Can you work these out from the model? Positions are in its coordinate system, mm. A direction names the side the tool comes from. Round coordinates to 2 decimals unless told otherwise and drop trailing zeros. Loops run counter-clockwise (first coordinate to the right, second up) from the corner with the lowest first, then second, coordinate; pieces in that order, holes last. Notation, with made-up numbers: M 58,69 L 105,69 A25 cw 105,95 Z; hole C 71,-31.75 d5. An arc over 180 degrees is marked long. Return JSON: item names as keys, results as strings.
```python
from build123d import *

# Parameters (mm, degrees)
IZIM1_R                     = 12.2
Y_KSEKLIK_EKSTR_ZYON1_DEPTH = 30.8
RADYUS1_R                   = 0.5
IZIM2_R                     = 12.2
Y_KSEKLIK_EKSTR_ZYON2_DEPTH = 21
IZIM3_R                     = 3.5
Y_KSEKLIK_EKSTR_ZYON3_DEPTH = 2.5
IZIM4_R                     = 2
Y_KSEKLIK_EKSTR_ZYON4_DEPTH = 9
IZIM5_R                     = 1
KES_EKSTR_ZYON1_DEPTH       = 10
IZIM6_R                     = 1.5
IZIM6_R_2                   = 1.3
KES_EKSTR_ZYON2_DEPTH       = 1
KES_EKSTR_ZYON3_START       = -8
KES_EKSTR_ZYON3_DEPTH       = 8
IZIM9_R                     = 3.25
Y_KSEKLIK_EKSTR_ZYON5_DEPTH = 1
IZIM10_R                    = 0.75
Y_KSEKLIK_EKSTR_ZYON6_DEPTH = 15
IZIM11_W                    = 0.852537123
IZIM11_H                    = 3
Y_KSEKLIK_EKSTR_ZYON7_DEPTH = 4
IZIM12_R                    = 0.75
KES_EKSTR_ZYON4_DEPTH       = 4
PAH1_SIZE                   = 1


with BuildPart() as part:
    # izim1 → Y_kseklik-Ekstr_zyon1 (new body)
    with BuildSketch(Plane.XY):
        with Locations(Location((-41.143471688, 10.161406423, 0), (0, 0, 180))):
            Circle(IZIM1_R)
    extrude(amount=Y_KSEKLIK_EKSTR_ZYON1_DEPTH)

    # Radyus1
    radyus1_edges = [part.edges().sort_by_distance(p)[0] for p in [
        (-28.943471688, 10.161406423, 30.8),
    ]]
    fillet(radyus1_edges, radius=RADYUS1_R)

    # izim2 → Y_kseklik-Ekstr_zyon2 (add)
    with BuildSketch(Plane.XY.offset(30.8)):
        with Locations(Location((-41.143471688, 10.161406423, 0), (0, 0, 180))):
            Circle(IZIM2_R)
    extrude(amount=Y_KSEKLIK_EKSTR_ZYON2_DEPTH)

    # izim3 → Y_kseklik-Ekstr_zyon3 (add)
    with BuildSketch(Plane.XY.offset(51.8)):
        with Locations((-41.143471688, 10.161406423)):
            Circle(IZIM3_R)
    extrude(amount=Y_KSEKLIK_EKSTR_ZYON3_DEPTH)

    # izim4 → Y_kseklik-Ekstr_zyon4 (add)
    with BuildSketch(Plane.XY.offset(54.3)):
        with Locations((-41.143471688, 10.161406423)):
            Circle(IZIM4_R)
    extrude(amount=Y_KSEKLIK_EKSTR_ZYON4_DEPTH)

    # izim5 → Kes-Ekstr_zyon1 (cut)
    with BuildSketch(Plane.XY.offset(51.8)):
        with Locations((-49.384663885, 10.161406423)):
            Circle(IZIM5_R)
        with Locations((-32.384663885, 10.161406423)):
            Circle(IZIM5_R)
    extrude(amount=-KES_EKSTR_ZYON1_DEPTH, mode=Mode.SUBTRACT)

    # izim6 → Kes-Ekstr_zyon2 (cut)
    # profile 1 of 4: a face of its own
    with BuildSketch(Plane.XY.offset(51.8)):
        with Locations((-41.143471688, 2.311406423)):
            Circle(IZIM6_R)
        with Locations((-41.143471688, 2.311406423)):
            Circle(IZIM6_R_2, mode=Mode.SUBTRACT)
    # profile 2 of 4: a face of its own
    with BuildSketch(Plane.XY.offset(51.8)):
        Polygon((-40.943471688, 1.311406423), (-40.943471688, 2.111406423), (-40.143471688, 2.111406423), (-40.143471688, 2.511406423), (-40.943471688, 2.511406423), (-40.943471688, 3.311406423), (-41.343471688, 3.311406423), (-41.343471688, 2.511406423), (-42.143471688, 2.511406423), (-42.143471688, 2.111406423), (-41.343471688, 2.111406423), (-41.343471688, 1.311406423), align=None)
    # profile 3 of 4: a face of its own
    with BuildSketch(Plane.XY.offset(51.8)):
        with Locations((-41.143471688, 18.011406423)):
            Circle(IZIM6_R)
        with Locations((-41.143471688, 18.011406423)):
            Circle(IZIM6_R_2, mode=Mode.SUBTRACT)
    # profile 4 of 4: a face of its own
    with BuildSketch(Plane.XY.offset(51.8)):
        Polygon((-41.343471688, 19.011406423), (-41.343471688, 18.211406423), (-42.143471688, 18.211406423), (-42.143471688, 17.811406423), (-41.343471688, 17.811406423), (-41.343471688, 17.011406423), (-40.943471688, 17.011406423), (-40.943471688, 17.811406423), (-40.143471688, 17.811406423), (-40.143471688, 18.211406423), (-40.943471688, 18.211406423), (-40.943471688, 19.011406423), align=None)
    extrude(amount=-KES_EKSTR_ZYON2_DEPTH, mode=Mode.SUBTRACT)

    # izim8 → Kes-Ekstr_zyon3 (cut)
    with BuildSketch(Plane.XY.offset(63.3).offset(KES_EKSTR_ZYON3_START)):
        with BuildLine():
            Line((-42.111717524, 11.911406423), (-40.175225851, 11.911406423))
            ThreePointArc((-40.175225851, 11.911406423), (-41.143471688, 12.161406423), (-42.111717524, 11.911406423))
        make_face()
    extrude(amount=KES_EKSTR_ZYON3_DEPTH, mode=Mode.SUBTRACT)

    # izim9 → Y_kseklik-Ekstr_zyon5 (add)
    with BuildSketch(Plane(origin=(0, 0, 0), x_dir=(-1, 0, 0), z_dir=(0, 0, -1))):
        with Locations(Location((41.143471688, 10.161406423, 0), (0, 0, 180))):
            Circle(IZIM9_R)
    extrude(amount=Y_KSEKLIK_EKSTR_ZYON5_DEPTH)

    # izim10 → Y_kseklik-Ekstr_zyon6 (add)
    with BuildSketch(Plane(origin=(0, 0, -1), x_dir=(-1, 0, 0), z_dir=(0, 0, -1))):
        with Locations(Location((41.143471688, 10.161406423, 0), (0, 0, 180))):
            Circle(IZIM10_R)
    extrude(amount=Y_KSEKLIK_EKSTR_ZYON6_DEPTH)

    # izim11 → Y_kseklik-Ekstr_zyon7 (add)
    with BuildSketch(Plane(origin=(0, 0, 0), x_dir=(-1, 0, 0), z_dir=(0, 0, -1))):
        with Locations((41.159259413, 18.661406423)):
            Rectangle(IZIM11_W, IZIM11_H)
        with Locations((41.159259413, 1.661406423)):
            Rectangle(IZIM11_W, IZIM11_H)
    extrude(amount=Y_KSEKLIK_EKSTR_ZYON7_DEPTH)

    # izim12 → Kes-Ekstr_zyon4 (cut)
    with BuildSketch(Plane(origin=(-40.732990851, 0, 0), x_dir=(0, 0, -1), z_dir=(1, 0, 0))):
        with Locations((1.925401768, 18.661406423)):
            Circle(IZIM12_R)
        with Locations((1.925401768, 1.661406423)):
            Circle(IZIM12_R)
    extrude(amount=-KES_EKSTR_ZYON4_DEPTH, mode=Mode.SUBTRACT)

    # Pah1
    pah1_edges = [part.edges().sort_by_distance(p)[0] for p in [
        (-41.159259412, 17.161406423, -4),
        (-41.159259412, 20.161406423, -4),
        (-41.159259412, 0.161406423, -4),
        (-41.159259412, 3.161406423, -4),
    ]]
    chamfer(pah1_edges, length=PAH1_SIZE)


solid = part.part
```
Q1. On a 3-axis mill with a long thin cutter (end or side, diameter ignored), from which of +Z, -Z, +X, -X, +Y, -Y can I reach the whole of each face in a straight line? I mean faces 4 (the cylindrical face through (-41.58, 8.21, 58.74)), 5 (the flat face through (-41.586, 19, -1)), 6 (the cylindrical face through (-28.955, 9.625, 41.153)), 7 (the cylindrical face through (-44.39, 10.02, -0.49)). Say none if no direction works.
Results:
{"face 4": "+Z", "face 5": "-Z, -X, +Y", "face 6": "+Z, -Z", "face 7": "-Z"}
Q2. Thinking about a two-plate mould opening in Z: for faces 1 (the flat face through (-41, 10, 63.3)), 2 (the cylindrical face through (-41.153, 17.996, -2.271)), 3 (the cylindrical face through (-40.8, 10.83, -8.4)), which applies, pulls with the +Z half, pulls with the -Z half, needs draft (parallel to the pull), parting line crosses it, or undercut?
Results:
{"face 1": "pulls with the +Z half", "face 2": "undercut", "face 3": "needs draft"}
Q3. I'm going to push flat-ended pins straight in: pin 1 Ø1.5 at (x, y) = (-39.5, 4) entering from -Z; pin 2 Ø1.8 at (x, y) = (-49.38, 10.16) entering from +Z; pin 3 Ø1 at (y, z) = (6.5, 0) entering from -X. Where does each tip first touch, or does it pass through?
Results:
{"pin 1": "stops at z = 0", "pin 2": "stops at z = 41.8", "pin 3": "stops at x = -52.93"}
Q4. If I drill on line 1 along Z through (x, y) = (-45.25, 21); line 2 along Y through (x, z) = (-35, 27); line 3 along X through (y, z) = (14.5, 1.5), over which ranges is the centre line in solid material (lowest first)?
Results:
{"line 1": "z = 0 to 51.8", "line 2": "y = -0.38 to 20.7", "line 3": "x = -52.55 to -29.74"}
Q5. Suppose I cut it at B-B, the plane z = 20. Please give me the cut outline in (x, y).
Results:
{"outline": "C -41.14,10.16 d24.4"}
Q6. Suppose I cut it at C-C, the plane z = -10. Please give me the cut outline in (x, y).
Results:
{"outline": "C -41.14,10.16 d1.5"}
Q7. Suppose I cut it at A-A, the plane z = 46. Please give me the cut outline in (x, y), plus the area to 3 significant figures.
Results:
{"outline": "C -41.14,10.16 d24.4; hole C -49.38,10.16 d2; hole C -32.38,10.16 d2", "area": "461 mm2"}
